Design review of the part built by this model. Coordinates are the model's own, in mm. A direction names the side the tool comes from. Coordinates: 2 decimals unless noted, no trailing zeros. Loops run counter-clockwise (first coordinate to the right, second up) from the corner with the lowest first, then second, coordinate; pieces in that order, holes last.
Q1. Add section C-C on x = -6.5. Give the boundary of the cut face in (y, z).
Q2. For P1, Ø1.5, axis at x = -27.5, z = 0, coming from the -Y side; P2, Ø6, axis at x = -46.5, z = 2.5, coming from the +Y side; P3, Ø0.8, axis at y = 0.5, z = -7, coming from the -X side; P4, Ø1.9, axis at x = -58.5, y = 3, coming from the -Z side, all flat-tipped, find the tip position at first contact; note any pin that passes through.
Q3. Machinability: for faces 1 (the face through (-52.388, 1, -8)), 2 (the face through (-52.388, 1, 8)), 3 (the face through (6.35, 0.78, 0.13)), which of the approach directions +Z, -Z, +X, -X, +Y, -Y give a long, thin tool a straight path to every point of the face, cutting with its end or side? Answer none if there is none.
Q4. Add section B-B on x = -31.75. Give the boundary of the cut face in (y, z), and give its area (3 significant figures).
Q5. Draft analysis for pull direction Z (two halves, no side actions). For faces 4 (the face through (-26.217, 0.783, 9.284)), 5 (the face through (-25.47, 0.78, -9.2)), 6 (the face through (-29.39, 0.78, 4.45)), state which applies: released by +Z, released by -Z, zero draft, split by the parting line, or undercut.
Q6. Wall thickness on probe 1 along Y at (x, z) = (-5.5, 6); probe 2 along Z at (x, y) = (-56, 1); probe 3 along X at (y, z) = (0.45, 0): over which ranges is each line inside the solid? List them lowest first.
Q7. Add section D-D on y = 5. Give the boundary of the cut face in (x, z), and give its area (3 significant figures).
```python
from build123d import *

# Parameters (mm, degrees)
SKETCH1_R               = 2.38125
BOSS_EXTRUDE1_DEPTH     = 1.5875
SKETCH2_W               = 25.4
SKETCH2_H               = 3.175
CUT_EXTRUDE1_DEPTH      = 62.831036149
CUT_EXTRUDE1_DEPTH_BACK = 62.831036149
SKETCH3_W               = 7.9375
SKETCH3_H               = 8.466666667


with BuildPart() as part:
    # Sketch1 → Boss-Extrude1 (new body)
    with BuildSketch(Plane(origin=(0, 0, 0), x_dir=(1, 0, 0), z_dir=(0, 1, 0))):
        with BuildLine():
            Line((-57.15, 12.7), (-57.15, -12.7))
            Line((-57.15, -12.7), (0.697028502, -6.311628258))
            ThreePointArc((0.697028502, -6.311628258), (6.35, 0), (0.697028502, 6.311628258))
            Line((0.697028502, 6.311628258), (-57.15, 12.7))
        make_face()
        with Locations(Location((0, 0, 0), (0, 0, 270))):
            Circle(SKETCH1_R, mode=Mode.SUBTRACT)
        with Locations(Location((-44.45, 6.35, 0), (0, 0, 270))):
            Circle(SKETCH1_R, mode=Mode.SUBTRACT)
        with Locations(Location((-31.75, -4.7625, 0), (0, 0, 270))):
            Circle(SKETCH1_R, mode=Mode.SUBTRACT)
    extrude(amount=BOSS_EXTRUDE1_DEPTH)

    # Sketch2 → Revolve1 (revolve)
    with BuildSketch(Plane.ZY.offset(57.15)):
        with Locations((0, 1.5875)):
            Rectangle(SKETCH2_W, SKETCH2_H)
    revolve(axis=Axis((-57.15, 3.175, -12.7), (0, 0, 1)))

    # Sketch3 → Cut-Extrude1 (cut, two sides: drawn at the far end of the back side and taken through both)
    with BuildSketch(Plane(origin=(0, 1.5875, 0), x_dir=(1, 0, 0), z_dir=(0, 1, 0)).offset(-CUT_EXTRUDE1_DEPTH_BACK)):
        with Locations((-56.35625, 8.466666667)):
            Rectangle(SKETCH3_W, SKETCH3_H)
        with Locations((-56.35625, -8.466666667)):
            Rectangle(SKETCH3_W, SKETCH3_H)
    extrude(amount=CUT_EXTRUDE1_DEPTH + CUT_EXTRUDE1_DEPTH_BACK, mode=Mode.SUBTRACT)


solid = part.part
```
Entries:
1. outline: (0, -7.11) - (1.59, -7.11) - (1.59, 7.11) - (0, 7.11) - close
2. P1: stops at y = 0
2. P2: stops at y = 1.59
2. P3: stops at x = -52.39
2. P4: stops at z = -4.23
3. face 1: -Z, -X, +Y, -Y
3. face 2: +Z, -X, +Y, -Y
3. face 3: +X, +Y, -Y
4. outline: (0, -9.89) - (1.59, -9.89) - (1.59, 2.38) - (0, 2.38) - close; (0, 7.14) - (1.59, 7.14) - (1.59, 9.89) - (0, 9.89) - close
4. area: 23.9 mm2
5. face 4: released by +Z
5. face 5: released by -Z
5. face 6: undercut
6. probe 1: y = 0 to 1.59
6. probe 2: z = -4.23 to 4.23
6. probe 3: x = -58.78 to -2.38, 2.38 to 6.35
7. outline: (-59.75, -4.23) - (-54.55, -4.23) - (-54.55, 4.23) - (-59.75, 4.23) - close
7. area: 44.0 mm2
